Read the model definition and answer for the solid it produces. Units are mm, in the model's axes. Face numbers are marked on the shaded views. A direction names the side the tool comes from. Give positions to 0.01 mm unless a question says otherwise; leave off trailing zeros. Loops run counter-clockwise (first coordinate to the right, second up) from the corner with the lowest first, then second, coordinate; pieces in that order, holes last. Notation, with made-up numbers: (84.25, 68.25) - (130.25, 68.25) arc R30 cw to (130.25, 104.25) - close; hole circle Ø7 at (-36.75, -17). An arc over 180 degrees is marked (long way). Write each question's results on one line, items separated by ' | '. Start each with the question number.
Q1. Given pin 1 (5 mm diameter, centred on x = -8.5, z = 12.5, fed in from -Y), flat-ended and moving along its own axis, determine where the tip first touches the part or whether it passes through.
Q2. Find the intervals of material crossed by line 1 (X direction, y = -1, z = 7.75); line 2 (X direction, y = 13.5, z = 2.75); line 3 (Y direction, x = 8.5, z = 7), in increasing order. Write a range as from..to.
Q3. Determine the mould class of the marked faces 1, 2 and 3 for opening direction X: +X half, -X half, draft (parallel to the pull), parting line (faces both ways), or undercut.
Q4. The part is cut by section A-A, the plane y = -0.5. Write down the section's boundary in (x, z), plus the area to 3 significant figures.
Q5. For the marked faces 4 and 5, determine the directions among +Z, -Z, +X, -X, +Y, -Y from which every point of the face is accessible in a straight line to the end or side of a thin tool.
Q6. The part is cut by section C-C, the plane x = -5. Write down the section's boundary in (y, z).
Q7. The part is cut by section D-D, the plane y = 13. Write down the section's boundary in (x, z).
Q8. The part is cut by section B-B, the plane z = 8.25. Write down the section's boundary in (x, y), plus the area to 3 significant figures.
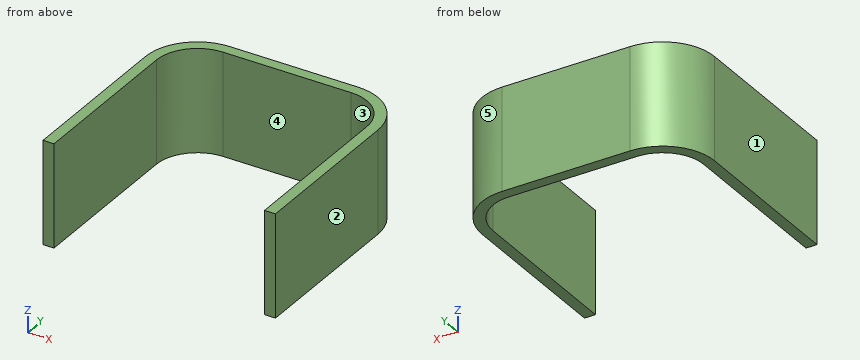
```python
from build123d import *

# Parameters (mm, degrees)
F1_DEPTH = 15
F2_R     = 6
F3_R     = 7.6


with BuildPart() as f1:
    # F0 (on Top) → F1 (new body)
    with BuildSketch(Plane.XY):
        Polygon((-16.95, -15.8), (-15.35, -15.8), (-15.35, 14.2), (15.35, 14.2), (15.35, -15.8), (16.95, -15.8), (16.95, 15.8), (-16.95, 15.8), align=None)
    extrude(amount=F1_DEPTH)

    # F2
    f2_edges = [f1.edges().sort_by_distance(p)[0] for p in [
        (-15.35, 14.2, 7.5),
        (15.35, 14.2, 7.5),
    ]]
    fillet(f2_edges, radius=F2_R)

    # F3
    f3_edges = [f1.edges().sort_by_distance(p)[0] for p in [
        (-16.95, 15.8, 7.5),
        (16.95, 15.8, 7.5),
    ]]
    fillet(f3_edges, radius=F3_R)


solid = f1.part
```
Check sheet entries:
1) pin 1: stops at y = 13.97
2) line 1: x = -16.95..-15.35, 15.35..16.95 | line 2: x = -14.8..-12.16, 12.16..14.8 | line 3: y = 14.2..15.8
3) face 1: -X half | face 2: +X half | face 3: undercut
4) outline: (-16.95, 0) - (-15.35, 0) - (-15.35, 15) - (-16.95, 15) - close; (15.35, 0) - (16.95, 0) - (16.95, 15) - (15.35, 15) - close | area: 48.0 mm^2
5) face 4: +Z, -Z, -Y | face 5: +Z, -Z, +X, +Y
6) outline: (14.2, 0) - (15.8, 0) - (15.8, 15) - (14.2, 15) - close
7) outline: (-15.24, 0) - (-12.95, 0) - (-12.95, 15) - (-15.24, 15) - close; (12.95, 0) - (15.24, 0) - (15.24, 15) - (12.95, 15) - close
8) outline: (-16.95, -15.8) - (-15.35, -15.8) - (-15.35, 8.2) arc R6 cw to (-9.35, 14.2) - (9.35, 14.2) arc R6 cw to (15.35, 8.2) - (15.35, -15.8) - (16.95, -15.8) - (16.95, 8.2) arc R7.6 ccw to (9.35, 15.8) - (-9.35, 15.8) arc R7.6 ccw to (-16.95, 8.2) - close | area: 141 mm^2
